```python
from build123d import *

# Parameters (mm, degrees)
SKETCH1_R               = 16
SKETCH1_R_2             = 6.6
BOSS_EXTRUDE1_DEPTH     = 43.5
SKETCH2_R               = 14
SKETCH2_R_2             = 10
BOSS_EXTRUDE2_DEPTH     = 14.5
SKETCH3_R               = 37.5
CUT_EXTRUDE1_DEPTH      = 17
CUT_EXTRUDE1_DEPTH_BACK = 17
BOSS_EXTRUDE3_REACH     = 60
SKETCH4_R               = 10
SKETCH4_R_2             = 6.6
SKETCH5_R               = 27.2
CUT_EXTRUDE2_DEPTH      = 17.0000001
CUT_EXTRUDE2_DEPTH_BACK = 17.0000001
CHAMFER1_SIZE           = 1


with BuildPart() as part:
    # Sketch1 → Boss-Extrude1 (new body)
    with BuildSketch(Plane(origin=(0, 0, 0), x_dir=(1, 0, 0), z_dir=(0, 1, 0))):
        Circle(SKETCH1_R)
        Circle(SKETCH1_R_2, mode=Mode.SUBTRACT)
    extrude(amount=BOSS_EXTRUDE1_DEPTH)

    # Sketch2 → Boss-Extrude2 (add)
    with BuildSketch(Plane(origin=(0, 43.5, 0), x_dir=(1, 0, 0), z_dir=(0, 1, 0))):
        Circle(SKETCH2_R)
        Circle(SKETCH2_R_2, mode=Mode.SUBTRACT)
    extrude(amount=BOSS_EXTRUDE2_DEPTH)

    # Sketch3 → Cut-Extrude1 (cut, two sides)
    with BuildSketch(Plane(origin=(0, 0, 0), x_dir=(0, 0, -1), z_dir=(1, 0, 0))) as cut_extrude1_sk:
        Circle(SKETCH3_R)
    extrude(amount=CUT_EXTRUDE1_DEPTH, mode=Mode.SUBTRACT)
    extrude(cut_extrude1_sk.sketch, amount=-CUT_EXTRUDE1_DEPTH_BACK, mode=Mode.SUBTRACT)

    # Sketch4 → Boss-Extrude3 (add, up to next)
    with BuildSketch(Plane(origin=(0, 0, 0), x_dir=(1, 0, 0), z_dir=(0, 1, 0)), mode=Mode.PRIVATE) as boss_extrude3_sk1:
        Circle(SKETCH4_R)
        Circle(SKETCH4_R_2, mode=Mode.SUBTRACT)
    boss_extrude3_tool1 = extrude(boss_extrude3_sk1.sketch, amount=BOSS_EXTRUDE3_REACH, mode=Mode.PRIVATE) - part.part
    add(boss_extrude3_tool1.solids().sort_by_distance((-9.717157, 0, 0))[0])

    # Sketch5 → Cut-Extrude2 (cut, two sides)
    with BuildSketch(Plane(origin=(0, 0, 0), x_dir=(0, 0, -1), z_dir=(1, 0, 0))) as cut_extrude2_sk:
        Circle(SKETCH5_R)
    extrude(amount=CUT_EXTRUDE2_DEPTH, mode=Mode.SUBTRACT)
    extrude(cut_extrude2_sk.sketch, amount=-CUT_EXTRUDE2_DEPTH_BACK, mode=Mode.SUBTRACT)

    # Chamfer1
    chamfer1_edges = [part.edges().sort_by_distance(p)[0] for p in [
        (-14, 58, 0),
    ]]
    chamfer(chamfer1_edges, length=CHAMFER1_SIZE)


solid = part.part
```
Read the model definition and answer for the solid it produces. Units are mm, in the model's axes. A direction names the side the tool comes from. Give positions to 0.01 mm unless a question says otherwise; leave off trailing zeros. Write each loop counter-clockwise with the first axis right and the second up, starting at its lowest first coordinate (ties: lowest second). Pieces come first, ordered by that corner, then holes. Notation, with made-up numbers: (32.25, 47.25) - (37.25, 47.25) arc R23 ccw to (37.25, 74.25) - close; hole circle Ø1 at (-36.75, -10). An arc over 180 degrees is marked (long way). Write item = value, one per line. Start each with the question number.
Item 1: A tool of negligible diameter and unlimited length cuts with its end or side. For faces 4 (the cylindrical face through (-15.985, 39.705, -0.703)), 5 (the cylindrical face through (-7.338, 36.827, 7.073)), 6 (the cylindrical face through (12.932, 50.156, 5.362)), from which of +Z, -Z, +X, -X, +Y, -Y can it reach the whole face along a straight path? Write none if from no direction.
Item 2: The mould has two halves that part along X. Classify faces 1 (the cylindrical face through (-2.17, 50.65, 9.76)), 2 (the cylindrical face through (-2.17, 31.32, 9.76)), 3 (the flat face through (7, 58, 8)): +X half, -X half, draft (parallel to the pull), parting line (faces both ways), or undercut.
Item 3: Find section A-A (z = 0). Give the vertices of the cut face in (x, y).
Item 4: Find section D-D (y = 35.5). Give the vertices of the cut face in (x, z), then the cut area to 3 significant figures.
Item 5: Find section C-C (y = 40). Give the vertices of the cut face in (x, z).
Item 6: Find the intervals of material crossed by probe 1 along Z at (x, y) = (0, 39); probe 2 along X at (y, z) = (31, 0), in increasing order. Write a range as [from, to].
Item 7: Each of these flat-tipped pins is pushed along its axis until it touches: P1, Ø12, axis at x = 0, z = 0, coming from the +Y side; P2, Ø6, axis at y = 44.5, z = -11.5, coming from the +X side; P3, Ø8, axis at x = -12.5, y = 36.5, coming from the -Z side; P4, Ø1.5, axis at x = 6, y = 50, coming from the -Z side. Where does it stop, or does it pass through?
Item 8: Find section B-B (x = 0). Give the vertices of the cut face in (y, z), then the cut area to 3 significant figures.
Response:
q1.face_4 = +Y, -Y
q1.face_5 = -Y
q1.face_6 = +Y
q2.face_1 = undercut
q2.face_2 = parting line
q2.face_3 = draft
q3.outline = (-16, 37.5) - (-10, 37.5) - (-10, 27.2) - (-6.6, 27.2) - (-6.6, 43.5) - (-10, 43.5) - (-10, 58) - (-13, 58) - (-14, 57) - (-14, 43.5) - (-16, 43.5) - close; (6.6, 27.2) - (10, 27.2) - (10, 37.5) - (16, 37.5) - (16, 43.5) - (14, 43.5) - (14, 57) - (13, 58) - (10, 58) - (10, 43.5) - (6.6, 43.5) - close
q4.outline = (-10.49, -12.08) arc R16 ccw to (10.49, -12.08) - close; (-10.49, 12.08) - (10.49, 12.08) arc R16 ccw to start; circle Ø20 at (0, 0); hole circle Ø13.2 at (0, 0)
q4.area = 290 mm²
q5.outline = circle Ø32 at (0, 0); hole circle Ø13.2 at (0, 0)
q6.probe_1 = [-16, -6.6], [6.6, 16]
q6.probe_2 = [-10, -6.6], [6.6, 10]
q7.P1 = through
q7.P2 = 13.45
q7.P3 = -13.56
q7.P4 = -12.98
q8.outline = (25.3, -10) - (36.14, -10) arc R37.5 cw to (33.92, -16) - (43.5, -16) - (43.5, -14) - (57, -14) - (58, -13) - (58, -10) - (43.5, -10) - (43.5, -6.6) - (26.39, -6.6) arc R27.2 cw to start; (25.3, 10) arc R27.2 cw to (26.39, 6.6) - (43.5, 6.6) - (43.5, 10) - (58, 10) - (58, 13) - (57, 14) - (43.5, 14) - (43.5, 16) - (33.92, 16) arc R37.5 cw to (36.14, 10) - close
q8.area = 335 mm²
